Autodesk Inventor part; units mm, degrees
ref_plane "YZ Plane" through (0, 0, 0) normal (1, 0, 0) x (0, 1, 0)
ref_plane "XZ Plane" through (0, 0, 0) normal (0, 1, 0) x (-1, 0, 0)
ref_plane "XY Plane" through (0, 0, 0) normal (0, 0, 1) x (1, 0, 0)
sketch "Sketch1" plane through (0, 0, 0) normal (0, 0, 1) x (1, 0, 0)
  line L0 (-174.625, 111.125) -> (130.175, 111.125)
  line L1 (130.175, 111.125) -> (130.175, -15.875)
  line L2 (130.175, -15.875) -> (-174.625, -15.875)
  line L3 (-174.625, -15.875) -> (-174.625, 111.125)
  point P0 (0, 0)
  dimension "d0" = 127
  dimension "d1" = 304.8
extrude "Extrusion1" add sketch "Sketch1" along normal blind 25.4
sketch "Sketch2" plane through (0, 0, 25.4) normal (0, 0, 1) x (1, 0, 0)
  arc A0 (-89.9147, 65.1281) -> (-91.28, 21.8576) centre (-105.641, 43.9675) ccw
  arc A1 (-91.3052, 80.8519) -> (-91.28, 7.0928) centre (-105.641, 43.9675) ccw
  arc A2 (-91.28, 7.0928) -> (-91.28, 21.8576) centre (-91.28, 14.4752) ccw
  arc A3 (-89.9147, 65.1281) -> (-91.3052, 80.8519) centre (-90.6099, 72.99) ccw
  line L0 (-69.1328, 16.3208) -> (-69.1328, 73.5344)
  line L1 (-54.368, 16.3208) -> (-54.368, 73.5344)
  arc A4 (-69.1328, 16.3208) -> (-54.368, 16.3208) centre (-61.7504, 14.4752) ccw
  arc A5 (-54.368, 73.5344) -> (-69.1328, 73.5344) centre (-61.7504, 73.5344) ccw
  arc A6 (-14.0573, 29.8688) -> (-54.368, 30.9892) centre (-34.5504, 18.2752) ccw
  arc A7 (-13.7648, 47.696) -> (-54.368, 47.696) centre (-34.0664, 34.6261) ccw
  line L2 (-14.0573, 29.8688) -> (-14.0573, 14.2776)
  line L3 (-14.0573, 48.1396) -> (-14.0573, 29.8688)
  line L4 (-30.3752, 14.2776) -> (-30.3752, 58.4872)
  arc A8 (-30.3752, 14.2776) -> (-14.0573, 14.2776) centre (-22.2162, 15.2758) ccw
  line L5 (2.8456, 15.2758) -> (2.8456, 58.4872)
  line L6 (21.3017, 15.2758) -> (21.3017, 58.4872)
  arc A9 (2.8456, 15.2758) -> (21.3017, 15.2758) centre (12.0736, 16.3458) ccw
  arc A10 (21.3017, 58.4872) -> (2.8456, 58.4872) centre (12.0736, 58.4872) ccw
  circle A11 centre (12.0736, 80.9168) radius 9.228
  circle A12 centre (68.1313, 53.8586) radius 21.2102
  circle A13 centre (68.1313, 53.8586) radius 8.0022
  arc A14 (49.3965, 3.6206) -> (89.1971, 33.323) centre (58.2137, 33.323) ccw
  line L7 (89.1971, 33.323) -> (89.1971, 51.3872)
  arc A15 (49.9069, 21.9732) -> (67.3833, 32.6616) centre (53.1362, 36.3249) ccw
  arc A16 (49.9069, 21.9732) -> (49.3965, 3.6206) centre (47.8533, 12.8469) ccw
  point P0 (0, 0)
  dimension "d42" = 13.208
  dimension "d43" = 13.208
emboss "Emboss1" sketch "Sketch2" operation cut depth 6.35 direction (0, 0, -1)
hole "Hole1" at (-163.3305, -4.0099, 25.4) direction (0, 0, -1) diameter 7.62 end through all
hole "Hole2" at (-163.7335, 100.3697, 25.4) direction (0, 0, -1) diameter 7.62 end through all
hole "Hole3" at (117.1647, 99.5637, 25.4) direction (0, 0, -1) diameter 7.62 end through all
hole "Hole4" at (117.5677, -6.025, 25.4) direction (0, 0, -1) diameter 7.62 end through all
properties part number "NewNameChirag"
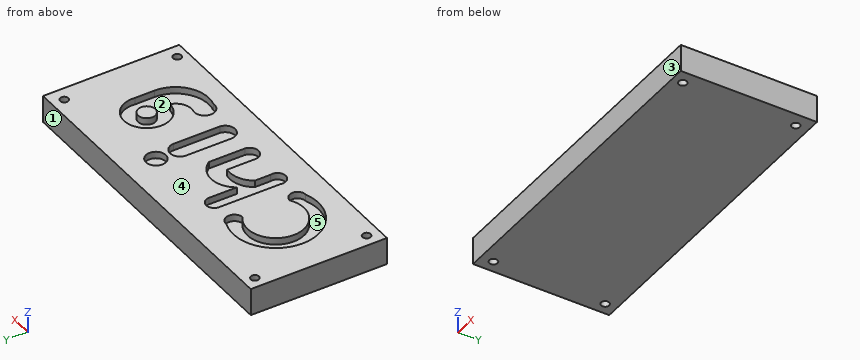
CAD build for the part. Positions are in the model's coordinates, mm. Face numbers are marked on the shaded views. A direction names the side the tool comes from. Give positions to 0.01 mm unless a question says otherwise; leave off trailing zeros. Put each result on its own line as item: value. Start each with the question number.
(1) Flat gauge pin, fed straight in: pin 1 Ø9 at (x, y) = (8, 30.5) entering from +Z. Where does the tip first touch, or does it go through?
(2) Probe L1, parallel to Y at x = 117, z = 23 (3 decimals); L2, parallel to X at y = 100, z = 4 (3 decimals); L3, parallel to X at y = -4, z = 14 (3 decimals). List the from-to ranges inside material, lowest first.
(3) Which spindle directions (+Z, -Z, +X, -X, +Y, -Y) get a long thin tool onto all of the face, cutting with end or side? Do the marked faces 4 and 5. Say none if no direction does.
(4) Mould opens along Y. For the marked faces 1, 2 and 3 say: +Y half, -Y half, draft (parallel to the pull), parting line (faces both ways), or undercut.
Response values:
1. pin 1: stops at z = 19.05
2. L1: y = -15.875 to -9.792, -2.258 to 95.757, 103.37 to 111.125
2. L2: x = -174.625 to -167.526, -159.941 to 113.38, 120.95 to 130.175
2. L3: x = -174.625 to -167.14, -159.521 to 114.34, 120.795 to 130.175
3. face 4: +Z, +X, -X, +Y, -Y
3. face 5: +Z
4. face 1: +Y half
4. face 2: undercut
4. face 3: -Y half
